Autodesk Inventor part; units mm, degrees
ref_plane "YZ Plane" through (0, 0, 0) normal (1, 0, 0) x (0, 1, 0)
ref_plane "XZ Plane" through (0, 0, 0) normal (0, 1, 0) x (-1, 0, 0)
ref_plane "XY Plane" through (0, 0, 0) normal (0, 0, 1) x (1, 0, 0)
sketch "Sketch1" plane through (0, 0, 0) normal (0, 1, 0) x (-1, 0, 0)
  circle A0 centre (9, 18) radius 1.6
  line L0 (0, 26.5631) -> (0, -32.5504)
  line L1 (19.3723, 0) -> (-25.4899, 0)
  circle A1 centre (9, -18) radius 1.6
  circle A2 centre (-9, 18) radius 1.6
  circle A3 centre (-9, -18) radius 1.6
  line L2 (13, 22) -> (-13, 22)
  line L3 (-13, 22) -> (-13, -22)
  line L4 (-13, -22) -> (13, -22)
  line L5 (13, -22) -> (13, 22)
  point P0 (0, 0)
  dimension "d0" = 3.2
  dimension "d3" = 36
  dimension "d6" = 18
  dimension "d9" = 4
  dimension "d10" = 4
extrude "Extrusion1" add sketch "Sketch1" along normal blind 3
sketch "Sketch2" plane through (13, 0, 22) normal (1, 0, 0) x (0, 0, -1)
  line L0 (0, 0) -> (44, 0)
  line L1 (44, 0) -> (44, 3)
  line L2 (0, 3) -> (44, 3)
  line L3 (0, 0) -> (0, 3)
  line L4 (0, 0) -> (44, 0)
  line L5 (8, 1.2) -> (36, 1.2)
  line L6 (36, 1.2) -> (36, 0)
  line L7 (36, 0) -> (8, 0)
  line L8 (8, 0) -> (8, 1.2)
  point P0 (22, 0)
  dimension "d13" = 1.2
  dimension "w" = 8
  dimension "d15" = 8
extrude "Extrusion2" cut sketch "Sketch2" against normal through all contours L8 L5 L6 L0
fillet "Fillet1" radius 1.2 2 edges at (0, 1.2, -14) (0, 1.2, 14)
equation "\"d15\" = w"
properties part number "piston-mount"
Work out the finished part from the listing and answer in its coordinate system (mm). A direction names the side the tool comes from. Round coordinates to 2 decimals unless told otherwise and drop trailing zeros. Loops run counter-clockwise (first coordinate to the right, second up) from the corner with the lowest first, then second, coordinate; pieces in that order, holes last. Notation, with made-up numbers: (-32, 33) - (21, 33) arc R22 cw to (21, 59) - close; hole circle Ø7 at (18.25, -16). An arc over 180 degrees is marked (long way). One line per item, written item: value.
Q1. Straight lines are drawn through the part: probe 1 along Z at (x, y) = (9, 1.55); probe 2 along Z at (x, y) = (-9, 0.95); probe 3 along Z at (x, y) = (7.75, 2.3). For each, find the intervals that lie inside material, in ascending order.
Check values:
probe 1: -22 to -19.6, -16.4 to 16.4, 19.6 to 22
probe 2: -22 to -19.6, -16.4 to -13.53, 13.53 to 16.4, 19.6 to 22
probe 3: -22 to -19, -17 to 17, 19 to 22
Q2. For faces 5 (the cylindrical face through (-8.792, 1.479, 16.414)), 6 (the flat face through (0, 1.2, 0)), determine the directions among +Z, -Z, +X, -X, +Y, -Y from which every point of the face is accessible in a straight line to the end or side of a thin tool.
Check values:
face 5: +Y, -Y
face 6: +X, -X, -Y
Q3. The mould has two halves that part along Z. Classify faces 1 (the flat face through (0, 3, 0)), 2 (the cylindrical face through (-0.18, 0.84, 13.66)), 3 (the flat face through (0, 1, 22)), 4 (the flat face through (0, 1, -22)): +Z half, -Z half, draft (parallel to the pull), parting line (faces both ways), or undercut.
Check values:
face 1: draft
face 2: undercut
face 3: +Z half
face 4: -Z half
Q4. Each of these flat-tipped pins is pushed along its axis until it touches: pin 1 Ø2 at (x, z) = (-7.5, 2.5) entering from -Y; pin 2 Ø4 at (x, z) = (9, 18) entering from +Y; pin 3 Ø1.9 at (x, z) = (-9, 18) entering from +Y. Where does it stop, or does it pass through?
Check values:
pin 1: y = 1.2
pin 2: y = 3
pin 3: through
Q5. Find section C-C on z = -18. Give the vertices of the cut face in (x, y), and give its area (3 significant figures).
Check values:
outline: (-13, 0) - (-10.6, 0) - (-10.6, 3) - (-13, 3) - close; (-7.4, 0) - (7.4, 0) - (7.4, 3) - (-7.4, 3) - close; (10.6, 0) - (13, 0) - (13, 3) - (10.6, 3) - close
area: 58.8 mm2
Q6. Find section B-B on x = 9. State how many separate pieces and enclosed holes the cut face has, and give its area (3 significant figures).
Check values:
separate pieces: 3
enclosed holes: 0
area: 79.8 mm2
Q7. Find section A-A on y = 1.7. Give the vertices of the cut face in (x, z).
Check values:
outline: (-13, -22) - (13, -22) - (13, 22) - (-13, 22) - close; hole circle Ø3.2 at (-9, -18); hole circle Ø3.2 at (-9, 18); hole circle Ø3.2 at (9, -18); hole circle Ø3.2 at (9, 18)
